```python
from build123d import *

# Parameters (mm, degrees)
F1_DEPTH       = 12.7
F2_R           = 12.7
F3_DEPTH       = 12.701
F4_SIZE        = 5.08
F6_D           = 4.4958
F6_CSINK_D     = 9.398
F6_CSINK_ANGLE = 82
F8_DEPTH       = 12.701
F10_DEPTH      = 3.81


with BuildPart() as f1:
    # F0 (on Front) → F1 (new body)
    with BuildSketch(Plane.XZ):
        with BuildLine():
            Line((112.346154, -35.169231), (127, 0))
            ThreePointArc((127, 0), (0, 25.4), (-127, 0))
            Line((-127, 0), (-112.346154, -35.169231))
            ThreePointArc((-112.346154, -35.169231), (0, -12.7), (112.346154, -35.169231))
        make_face()
    extrude(amount=F1_DEPTH)

    # F2 (on face) → F3 (cut, through all)
    with BuildSketch(Plane.XZ.offset(12.7)):
        with Locations((61.094761, 0.293023)):
            Circle(F2_R)
        with Locations((-89.780517, -6.884272)):
            Circle(F2_R)
        with Locations((10.635643, 6.168175)):
            Circle(F2_R)
        with Locations((-40.106974, 3.754295)):
            Circle(F2_R)
    extrude(amount=-F3_DEPTH, mode=Mode.SUBTRACT)

    # F4
    f4_edges = [f1.edges().sort_by_distance(p)[0] for p in [
        (-119.673077, -12.7, -17.584615),
        (119.673077, -12.7, -17.584615),
    ]]
    chamfer(f4_edges, length=F4_SIZE)

    # F6 (through all)
    with Locations(Plane.XZ.offset(12.7)):
        with Locations((-6.879248, -1.323894), (28.150535, 13.660243), (43.655768, -7.374051), (78.533754, 7.960097), (-77.058188, 7.294757), (-102.502846, -21.0633), (-54.807347, -8.361872), (-25.4066, 15.870463)):
            CounterSinkHole(F6_D / 2, F6_CSINK_D / 2, counter_sink_angle=F6_CSINK_ANGLE)

    # F7 (on face) → F8 (cut, through all)
    with BuildSketch(Plane.XZ.offset(12.7)):
        with BuildLine():
            ThreePointArc((104.981769, -15.270498), (109.048898, -13.367943), (107.146343, -9.300814))
            ThreePointArc((107.146343, -9.300814), (98.050229, -6.159313), (88.86221, -3.297736))
            ThreePointArc((88.86221, -3.297736), (84.919132, -5.445616), (87.067013, -9.388694))
            ThreePointArc((87.067013, -9.388694), (96.069415, -12.192461), (104.981769, -15.270498))
        make_face()
    extrude(amount=-F8_DEPTH, mode=Mode.SUBTRACT)

    # F9 (on face) → F10 (cut)
    with BuildSketch(Plane.XZ.offset(12.7)):
        with BuildLine():
            ThreePointArc((108.012172, -6.912941), (98.842554, -3.746053), (89.580289, -0.861353))
            ThreePointArc((89.580289, -0.861353), (82.482749, -4.727538), (86.348934, -11.825077))
            ThreePointArc((86.348934, -11.825077), (95.27709, -14.60572), (104.11594, -17.658371))
            ThreePointArc((104.11594, -17.658371), (111.436771, -14.233772), (108.012172, -6.912941))
        make_face()
        with BuildLine():
            ThreePointArc((88.86221, -3.297736), (98.050229, -6.159313), (107.146343, -9.300814))
            ThreePointArc((107.146343, -9.300814), (109.048898, -13.367943), (104.981769, -15.270498))
            ThreePointArc((104.981769, -15.270498), (96.069415, -12.192461), (87.067013, -9.388694))
            ThreePointArc((87.067013, -9.388694), (84.919132, -5.445616), (88.86221, -3.297736))
        make_face(mode=Mode.SUBTRACT)
    extrude(amount=-F10_DEPTH, mode=Mode.SUBTRACT)


solid = f1.part
```
Geometry: final body of the model. Coordinates: model frame, mm. A direction names the side the tool comes from. Coordinates: 2 decimals unless noted, no trailing zeros. Order: outer loops, then holes, each group sorted by start corner. A loop starts at its lowest first (then second) coordinate and runs counter-clockwise, first axis right, second up. Notation, with made-up numbers: M -22.5,-13.5 L 0.5,-13.5 A20 cw 0.5,20.5 Z; hole C -15,48.25 d5. An arc over 180 degrees is marked long. Answer in a Markdown table with one row per item. Add a question column.
Q1. Section query D-D on x = 97. Return the cut outline in (y, z).
Q2. Contact query for flat-ended pins moving along their axis: P1, Ø5, axis at x = -102.5, z = -21.06, coming from the -Y side; P2, Ø6, axis at x = -77.06, z = 7.29, coming from the -Y side; P3, Ø3, axis at x = 76, y = -3.5, coming from the +Z side. Output: stop coordinate, or through.
Q3. Section query A-A on x = 5. Return the cut outline in (y, z), and give its area (3 significant figures).
Q4. Section query C-C on x = 55. Return the cut outline in (y, z).
Q5. Mould query, pull axis Z, two halves, no side actions, for faces 3 (the cylindrical face through (73.208, -6.439, 4.108)), 4 (the flat face through (-119.776, -3.757, -17.338)), 5 (the cylindrical face through (1.825, -6.261, 25.395)). Classes: released by +Z, released by -Z, zero draft, split by the parting line, or undercut.
Q6. Section query B-B on y = -3.75. Count the separate pieces of the cut face and the enclosed holes in it, and give its area (3 significant figures).
Q7. Line query: L1, parallel to Z at x = 61, y = -4.75; L2, parallel to X at y = -1.75, z = 0; L3, parallel to Z at x = 80.5, y = -1.5. Output: solid intervals per line, ascending.
Q8. Reachability of faces 1 (the cylindrical face through (95.94, -4.51, -12.15)), 2 (the cylindrical face through (82.52, -10.82, -4.61)) from +Z, -Z, +X, -X, +Y, -Y: full face, straight path, thin tool, end or side. Return the list, or none.
Completed:
| question | item | result |
|---|---|---|
| 1 | outline | M -12.7,-29.28 L 0,-29.28 L 0,-12.5 L -8.89,-12.5 L -8.89,-15.18 L -12.7,-15.18 Z; M -12.7,-3.15 L -8.89,-3.15 L -8.89,-5.82 L 0,-5.82 L 0,10.83 L -12.7,10.83 Z |
| 2 | P1 | stops at y = -10.18 |
| 2 | P2 | stops at y = -10.75 |
| 2 | P3 | stops at z = 16.89 |
| 3 | outline | M -12.7,-12.74 L 0,-12.74 L 0,-5.21 L -12.7,-5.21 Z; M -12.7,17.55 L 0,17.55 L 0,25.36 L -12.7,25.36 Z |
| 3 | area | 195 mm2 |
| 4 | outline | M -12.7,-17.92 L 0,-17.92 L 0,-10.85 L -12.7,-10.85 Z; M -12.7,11.44 L 0,11.44 L 0,20.79 L -12.7,20.79 Z |
| 5 | face 3 | undercut |
| 5 | face 4 | released by -Z |
| 5 | face 5 | released by +Z |
| 6 | separate pieces | 1 |
| 6 | enclosed holes | 13 |
| 6 | area | 7,050 mm2 |
| 7 | L1 | z = -19.14 to -12.41, 12.99 to 19.72 |
| 7 | L2 | x = -127 to -100.45, -79.11 to -52.24, -27.97 to -8.7, -5.06 to -0.47, 21.74 to 48.4, 73.79 to 127 |
| 7 | L3 | z = -24.01 to 6.87, 9.05 to 15.44 |
| 8 | face 1 | +Y, -Y |
| 8 | face 2 | -Y |
